```python
from build123d import *

# Parameters (mm, degrees)
CUT_EXTRUDE2_DEPTH      = 198.226946435
CUT_EXTRUDE2_DEPTH_BACK = 198.226946435
SKETCH3_W               = 77.6
SKETCH3_H               = 9.49


with BuildPart() as part:
    # Sketch1 → Revolve2 (revolve)
    with BuildSketch(Plane.XY, mode=Mode.PRIVATE) as revolve2_sk:
        Polygon((191.14, 0), (191.14, 14.37), (161.14, 14.37), (161.14, 19.73), (24.76, 19.73), (24.76, 34.38), (0, 34.38), (0, 18.68), (142.46, 18.68), (142.46, 0), align=None)
    revolve(revolve2_sk.sketch.rotate(Axis((0, 0, 0), (1, 0, 0)), 180), axis=Axis((0, 0, 0), (1, 0, 0)))

    # Sketch3 → Cut-Extrude2 (cut, two sides: drawn at the far end of the back side and taken through both)
    with BuildSketch(Plane(origin=(0, 0, 0), x_dir=(1, 0, 0), z_dir=(0, 1, 0)).offset(-CUT_EXTRUDE2_DEPTH_BACK)):
        with Locations((63.56, 0)):
            Rectangle(SKETCH3_W, SKETCH3_H)
    extrude(amount=CUT_EXTRUDE2_DEPTH + CUT_EXTRUDE2_DEPTH_BACK, mode=Mode.SUBTRACT)


solid = part.part
```
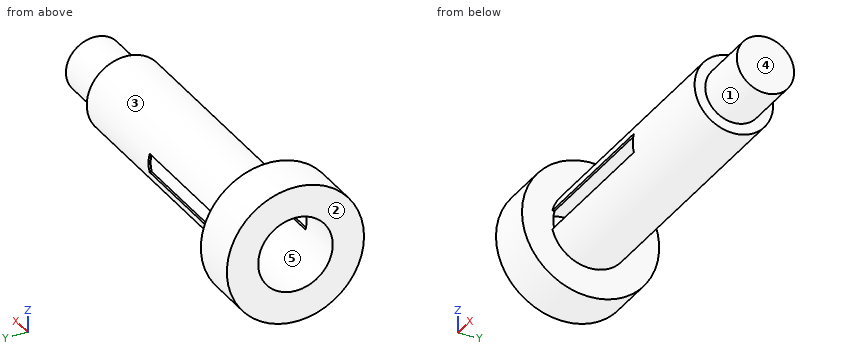
Geometry check sheet. Reference: the model listing, model coordinates, mm. Face numbers are marked on the shaded views. A direction names the side the tool comes from. Round coordinates to 2 decimals unless told otherwise and drop trailing zeros. Loops run counter-clockwise (first coordinate to the right, second up) from the corner with the lowest first, then second, coordinate; pieces in that order, holes last. Notation, with made-up numbers: M 27,5 L 75,5 A21 ccw 75,13 Z; hole C 78.5,73.5 d8. An arc over 180 degrees is marked long. Return JSON: item names as keys, results as strings. Group by question number.
(1) Section check C-C, the plane y = -11.5. Enter the section's corners in (x, z), and give its area (3 significant figures).
(2) Section check D-D, the plane x = 23. Enter the section's corners in (y, z), and give its area (3 significant figures).
(3) Section check A-A, the plane z = 0. Enter the section's corners in (x, y).
(4) Section check B-B, the plane x = 57. Enter the section's corners in (y, z) (3 decimals).
(5) Mould release check, pull along Z, two halves, no side actions. Record for the marked faces 3, 4 and 5: pulls with the +Z half, pulls with the -Z half, needs draft (parallel to the pull), parting line crosses it, or undercut.
(6) Scan lines: line 1 along Z through (x, y) = (58, 0); line 2 along X through (y, z) = (6, 2.5); line 3 along X through (y, z) = (-4.5, -21). Record each from-to range of solid material in increasing order. Write a range as [from, to].
(7) Set-up check for the marked faces 1 and 2: record each of +Z, -Z, +X, -X, +Y, -Y from which the full face is reachable in a straight line by a thin tool's end or side.
(8) Go/stop test with flat-tipped pins: pin 1 (1.3 mm diameter, centred on y = 19, z = 0.5, fed in from -X); pin 2 (6 mm diameter, centred on x = 55, z = 3, fed in from +Y); pin 3 (12 mm diameter, centred on x = 143.5, y = 13, fed in from -Z); pin 4 (8 mm diameter, centred on x = 85, z = 26.5, fed in from +Y). Record where each tip stops, or that it passes through.
Data:
{
 "1": {"outline": "M 0,-32.4 L 24.76,-32.4 L 24.76,-16.03 L 161.14,-16.03 L 161.14,-8.62 L 191.14,-8.62 L 191.14,8.62 L 161.14,8.62 L 161.14,16.03 L 24.76,16.03 L 24.76,32.4 L 0,32.4 L 0,14.72 L 142.46,14.72 L 142.46,-14.72 L 0,-14.72 Z", "area": "2,300 mm²"},
 "2": {"outline": "C 0,0 d68.76; hole C 0,0 d37.36", "area": "2,620 mm²"},
 "3": {"outline": "M 0,-34.38 L 24.76,-34.38 L 24.76,-18.68 L 0,-18.68 Z; M 0,18.68 L 24.76,18.68 L 24.76,34.38 L 0,34.38 Z; M 102.36,-19.73 L 161.14,-19.73 L 161.14,-14.37 L 191.14,-14.37 L 191.14,14.37 L 161.14,14.37 L 161.14,19.73 L 102.36,19.73 L 102.36,18.68 L 142.46,18.68 L 142.46,-18.68 L 102.36,-18.68 Z"},
 "4": {"outline": "M -19.151,-4.745 A19.73 ccw 19.151,-4.745 L 18.067,-4.745 A18.68 cw -18.067,-4.745 Z; M -19.151,4.745 L -18.067,4.745 A18.68 cw 18.067,4.745 L 19.151,4.745 A19.73 ccw Z"},
 "5": {"face 3": "parting line crosses it", "face 4": "needs draft", "face 5": "undercut"},
 "6": {"line 1": "[-19.73, -18.68], [18.68, 19.73]", "line 2": "[142.46, 191.14]", "line 3": "[0, 24.76]"},
 "7": {"face 1": "+X", "face 2": "+Z, -Z, -X, +Y, -Y"},
 "8": {"pin 1": "x = 0", "pin 2": "y = 19.15", "pin 3": "z = -18.45", "pin 4": "through"}
}
